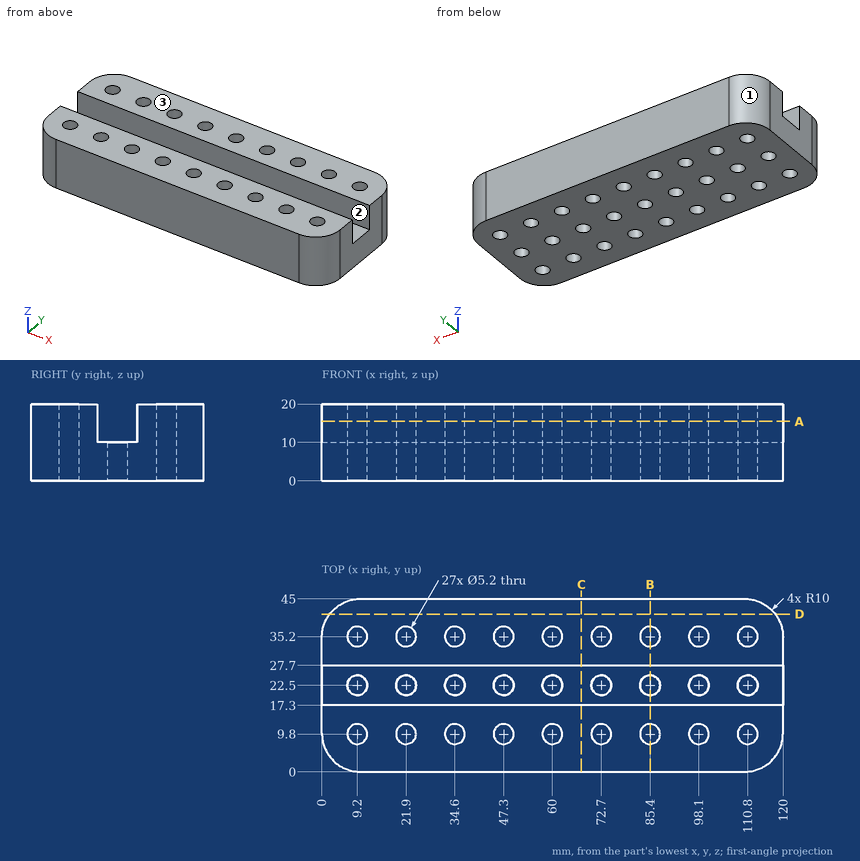
Part print with two shaded views. Sizes in mm from the minimum x, y, z corner. Coordinates: 2 decimals unless noted, no trailing zeros. Order: outer loops, then holes, each group sorted by start corner. A loop starts at its lowest first (then second) coordinate and runs counter-clockwise, first axis right, second up. Notation, with made-up numbers: (47, 19.25) - (53, 19.25) arc R31 cw to (53, 53.25) - close; hole circle Ø4 at (-37, 25). An arc over 180 degrees is marked (long way). Write item = value, one per line. Start each with the question number.
1) Saw through at A-A on z = 15.5. Count the separate pieces of the cut face and the enclosed holes in it, then the cut area to 3 significant figures.
2) Saw through at C-C on x = 67.5. Write the cut outline in (y, z), then the cut area to 3 significant figures.
3) Wall check: line 1 along Y through (x, z) = (21.9, 13.75); line 2 along Y through (x, z) = (47.5, 5.75); line 3 along Y through (x, z) = (106, 12.75). Give the ranges that are in metal, low to high. Write a range as from..to.
4) Flat gauge pins, fed straight in: pin 1 Ø2 at (y, z) = (37.5, 7.5) entering from -X; pin 2 Ø1 at (y, z) = (5, 17) entering from +X; pin 3 Ø6 at (x, y) = (85.4, 22.5) entering from +Z. Where does each tip first touch, or does it go through?
5) Saw through at D-D on y = 41. Write the cut outline in (x, z), then the cut area to 3 significant figures.
6) Saw through at B-B on x = 85.4. Write the cut outline in (y, z), then the cut area to 3 significant figures.
7) Two-plate mould, pull along Y, no slides. Class the marked faces 1, 2 and 3: pulls with the +Y half, pulls with the -Y half, needs draft (parallel to the pull), parting line crosses it, or undercut.
From the geometry:
q1.separate_pieces = 2
q1.enclosed_holes = 18
q1.area = 3,680 mm^2
q2.outline = (0, 0) - (45, 0) - (45, 20) - (27.7, 20) - (27.7, 10) - (17.3, 10) - (17.3, 20) - (0, 20) - close
q2.area = 796 mm^2
q3.line_1 = 0..7.2, 12.4..17.3, 27.7..32.6, 37.8..45
q3.line_2 = 0..7.21, 12.39..19.91, 25.09..32.61, 37.79..45
q3.line_3 = 0..17.3, 27.7..45
q4.pin_1 = 0.11
q4.pin_2 = 118.93
q4.pin_3 = 10
q5.outline = (2, 0) - (118, 0) - (118, 20) - (2, 20) - close
q5.area = 2,320 mm^2
q6.outline = (0, 0) - (7.2, 0) - (7.2, 20) - (0, 20) - close; (12.4, 0) - (19.9, 0) - (19.9, 10) - (17.3, 10) - (17.3, 20) - (12.4, 20) - close; (25.1, 0) - (32.6, 0) - (32.6, 20) - (27.7, 20) - (27.7, 10) - (25.1, 10) - close; (37.8, 0) - (45, 0) - (45, 20) - (37.8, 20) - close
q6.area = 536 mm^2
q7.face_1 = pulls with the +Y half
q7.face_2 = undercut
q7.face_3 = needs draft
